Part model, mm, in its own coordinate system. A direction names the side the tool comes from. Round coordinates to 2 decimals unless told otherwise and drop trailing zeros. Write each loop counter-clockwise with the first axis right and the second up, starting at its lowest first coordinate (ties: lowest second). Pieces come first, ordered by that corner, then holes. Notation, with made-up numbers: (-26.5, 61.25) -> (8.5, 61.25) arc R27 cw to (8.5, 91.25) -> close; hole circle Ø10 at (-11, 66). An arc over 180 degrees is marked (long way). Return JSON: item names as keys, results as strings. Group by question number.
```python
from build123d import *

# Parameters (mm, degrees)
BOSS_EXTRUDE1_DEPTH     = 12.88
SWEEP1_START            = 0.63
SWEEP1_DEPTH            = 1.52
LPATTERN1_COUNT         = 3
LPATTERN1_PITCH         = 5
SKETCH5_W               = 2.9
SKETCH5_H               = 0.8
CUT_EXTRUDE1_DEPTH      = 1
LPATTERN2_COUNT         = 2
LPATTERN2_PITCH         = 5.58
MIRROR1_START           = 0.63
MIRROR1_COPY_1_DEPTH    = 1.52
MIRROR1_COPY_2_DEPTH    = 1.52
MIRROR1_COPY_3_SKETCH_W = 2.9
MIRROR1_COPY_3_SKETCH_H = 0.8
MIRROR1_COPY_3_DEPTH    = 1
CUT_EXTRUDE2_REACH      = 21.386
SKETCH6_R               = 1.8
SKETCH7_R               = 2.2
SKETCH7_R_2             = 1.8
BOSS_EXTRUDE2_DEPTH     = 1.4
CUT_EXTRUDE3_DEPTH      = 17.621667755


# Read off the part's stored shape, not the designer's step: Sweep1
with BuildPart() as part:
    # Sketch1 → Boss-Extrude1 (new body)
    with BuildSketch(Plane(origin=(0, 0, 0), x_dir=(0, 0, -1), z_dir=(1, 0, 0))):
        with BuildLine():
            Line((0, 0), (0, 5.15))
            ThreePointArc((0, 5.15), (0.351471863, 5.998528137), (1.2, 6.35))
            Line((1.2, 6.35), (6.7, 6.35))
            ThreePointArc((6.7, 6.35), (7.548528137, 5.998528137), (7.9, 5.15))
            Line((7.9, 5.15), (7.9, 0))
            Line((7.9, 0), (7.1, 0))
            Line((7.1, 0), (7.1, 5.15))
            ThreePointArc((7.1, 5.15), (6.982842712, 5.432842712), (6.7, 5.55))
            Line((6.7, 5.55), (1.2, 5.55))
            ThreePointArc((1.2, 5.55), (0.917157288, 5.432842712), (0.8, 5.15))
            Line((0.8, 5.15), (0.8, 0))
            Line((0.8, 0), (0, 0))
        make_face()
    extrude(amount=BOSS_EXTRUDE1_DEPTH)

    # Sweep1 outline → Sweep1 (add)
    with BuildSketch(Plane.YZ.offset(SWEEP1_START)):
        with BuildLine():
            add(Edge.make_bspline(
                [(-0.846283759, -8.124029358), (-0.858016898, -8.129757785), (-0.870152204, -8.135642842), (-1.003345202, -8.19967658), (-1.15196737, -8.253874655), (-1.433217357, -8.328196696), (-1.577221625, -8.352525408), (-2.012213537, -8.385830326), (-2.305250753, -8.352541538), (-2.584692284, -8.272379972)],
                knots=[-0.008659355, -0.008659355, -0.008659355, -0.008659355, 0, 0, 0.081660017, 0.081660017, 0.163320034, 0.163320034, 0.326640068, 0.326640068, 0.326640068, 0.326640068], degree=3))
            ThreePointArc((-0.846283759, -8.124029358), (-0.431086788, -7.982015265), (0, -7.9))
            Line((0, -7.9), (0, -7.1))
            add(Edge.make_bspline(
                [(0, -7.1), (-0.377073857, -7.135252748), (-0.796992874, -7.239007705), (-1.153651992, -7.390208706), (-1.166116228, -7.395524363), (-1.178338095, -7.400759688)],
                knots=[0, 0, 0, 0, 1, 1, 1.037382886, 1.037382886, 1.037382886, 1.037382886], degree=3))
            ThreePointArc((-1.178338095, -7.400759688), (-1.724000867, -7.564826814), (-2.292574798, -7.527620028))
            Line((-2.292574798, -7.527620028), (-5.183941257, -6.727620028))
            Line((-5.183941257, -6.727620028), (-5.476058743, -7.472379972))
            Line((-5.476058743, -7.472379972), (-2.584692284, -8.272379972))
        make_face()
    sweep1 = extrude(amount=SWEEP1_DEPTH)

    # LPattern1: Sweep1 ×3
    with Locations(*[(i * LPATTERN1_PITCH, 0, 0) for i in range(1, LPATTERN1_COUNT)]):
        add(sweep1)

    # Sketch5 → Cut-Extrude1 (cut)
    with BuildSketch(Plane.XZ):
        with Locations((3.6, -7.5)):
            Rectangle(SKETCH5_W, SKETCH5_H)
    cut_extrude1 = extrude(amount=-CUT_EXTRUDE1_DEPTH, mode=Mode.SUBTRACT)

    # LPattern2: Cut-Extrude1 ×2
    with Locations(*[(i * LPATTERN2_PITCH, 0, 0) for i in range(1, LPATTERN2_COUNT)]):
        add(cut_extrude1, mode=Mode.SUBTRACT)

    # Mirror1: Sweep1, Cut-Extrude1 across plane
    add(sweep1.mirror(Plane(origin=(0, 0, -3.95), x_dir=(1, 0, 0), z_dir=(0, 0, -1))))
    add(cut_extrude1.mirror(Plane(origin=(0, 0, -3.95), x_dir=(1, 0, 0), z_dir=(0, 0, -1))), mode=Mode.SUBTRACT)

    # Mirror1 copy 1 sketch → Mirror1 copy 1 (add)
    with BuildSketch(Plane(origin=(5, 0, -7.9), x_dir=(0, 1, 0), z_dir=(1, 0, 0)).offset(MIRROR1_START)):
        with BuildLine():
            add(Edge.make_bspline(
                [(-0.846283759, 8.124029358), (-0.858016898, 8.129757785), (-0.870152204, 8.135642842), (-1.003345202, 8.19967658), (-1.15196737, 8.253874655), (-1.433217357, 8.328196696), (-1.577221625, 8.352525408), (-2.012213537, 8.385830326), (-2.305250753, 8.352541538), (-2.584692284, 8.272379972)],
                knots=[-0.008659355, -0.008659355, -0.008659355, -0.008659355, 0, 0, 0.081660017, 0.081660017, 0.163320034, 0.163320034, 0.326640068, 0.326640068, 0.326640068, 0.326640068], degree=3))
            ThreePointArc((-0.846283759, 8.124029358), (-0.431086788, 7.982015265), (0, 7.9))
            Line((0, 7.9), (0, 7.1))
            add(Edge.make_bspline(
                [(0, 7.1), (-0.377073857, 7.135252748), (-0.796992874, 7.239007705), (-1.153651992, 7.390208706), (-1.166116228, 7.395524363), (-1.178338095, 7.400759688)],
                knots=[0, 0, 0, 0, 1, 1, 1.037382886, 1.037382886, 1.037382886, 1.037382886], degree=3))
            ThreePointArc((-1.178338095, 7.400759688), (-1.724000867, 7.564826814), (-2.292574798, 7.527620028))
            Line((-2.292574798, 7.527620028), (-5.183941257, 6.727620028))
            Line((-5.183941257, 6.727620028), (-5.476058743, 7.472379972))
            Line((-5.476058743, 7.472379972), (-2.584692284, 8.272379972))
        make_face()
    extrude(amount=MIRROR1_COPY_1_DEPTH)

    # Mirror1 copy 2 sketch → Mirror1 copy 2 (add)
    with BuildSketch(Plane(origin=(10, 0, -7.9), x_dir=(0, 1, 0), z_dir=(1, 0, 0)).offset(MIRROR1_START)):
        with BuildLine():
            add(Edge.make_bspline(
                [(-0.846283759, 8.124029358), (-0.858016898, 8.129757785), (-0.870152204, 8.135642842), (-1.003345202, 8.19967658), (-1.15196737, 8.253874655), (-1.433217357, 8.328196696), (-1.577221625, 8.352525408), (-2.012213537, 8.385830326), (-2.305250753, 8.352541538), (-2.584692284, 8.272379972)],
                knots=[-0.008659355, -0.008659355, -0.008659355, -0.008659355, 0, 0, 0.081660017, 0.081660017, 0.163320034, 0.163320034, 0.326640068, 0.326640068, 0.326640068, 0.326640068], degree=3))
            ThreePointArc((-0.846283759, 8.124029358), (-0.431086788, 7.982015265), (0, 7.9))
            Line((0, 7.9), (0, 7.1))
            add(Edge.make_bspline(
                [(0, 7.1), (-0.377073857, 7.135252748), (-0.796992874, 7.239007705), (-1.153651992, 7.390208706), (-1.166116228, 7.395524363), (-1.178338095, 7.400759688)],
                knots=[0, 0, 0, 0, 1, 1, 1.037382886, 1.037382886, 1.037382886, 1.037382886], degree=3))
            ThreePointArc((-1.178338095, 7.400759688), (-1.724000867, 7.564826814), (-2.292574798, 7.527620028))
            Line((-2.292574798, 7.527620028), (-5.183941257, 6.727620028))
            Line((-5.183941257, 6.727620028), (-5.476058743, 7.472379972))
            Line((-5.476058743, 7.472379972), (-2.584692284, 8.272379972))
        make_face()
    extrude(amount=MIRROR1_COPY_2_DEPTH)

    # Mirror1 copy 3 sketch → Mirror1 copy 3 (cut)
    with BuildSketch(Plane(origin=(5.58, 0, -7.9), x_dir=(1, 0, 0), z_dir=(0, -1, 0))):
        with Locations((3.6, 7.5)):
            Rectangle(MIRROR1_COPY_3_SKETCH_W, MIRROR1_COPY_3_SKETCH_H)
    extrude(amount=-MIRROR1_COPY_3_DEPTH, mode=Mode.SUBTRACT)

    # Sketch6 → Cut-Extrude2 (cut, up to next)
    with BuildSketch(Plane(origin=(0, 6.35, 0), x_dir=(1, 0, 0), z_dir=(0, 1, 0)), mode=Mode.PRIVATE) as cut_extrude2_sk1:
        with Locations(Location((6.44, 3.95, 0), (0, 0, 270))):
            Circle(SKETCH6_R)
    cut_extrude2_tool1 = extrude(cut_extrude2_sk1.sketch, amount=-CUT_EXTRUDE2_REACH, mode=Mode.PRIVATE) & part.part
    add(cut_extrude2_tool1.solids().sort_by_distance((6.44, 6.35, -3.95))[0], mode=Mode.SUBTRACT)

    # Sketch7 → Boss-Extrude2 (add)
    with BuildSketch(Plane.XZ.offset(-5.55)):
        with Locations(Location((6.44, -3.95, 0), (0, 0, 90))):
            Circle(SKETCH7_R)
        with Locations(Location((6.44, -3.95, 0), (0, 0, 90))):
            Circle(SKETCH7_R_2, mode=Mode.SUBTRACT)
    extrude(amount=BOSS_EXTRUDE2_DEPTH)

    # Sketch8 → Cut-Extrude3 (cut, through all)
    with BuildSketch(Plane.ZY):
        Polygon((-6.603043073, 6.35), (-6.453043073, 6.2), (-6.303043073, 6.35), align=None)
        Polygon((-5.303043073, 6.35), (-5.603043073, 6.35), (-5.453043073, 6.2), align=None)
        Polygon((-4.303043073, 6.35), (-4.603043073, 6.35), (-4.453043073, 6.2), align=None)
        Polygon((-3.303043073, 6.35), (-3.603043073, 6.35), (-3.453043073, 6.2), align=None)
        Polygon((-2.303043073, 6.35), (-2.603043073, 6.35), (-2.453043073, 6.2), align=None)
        Polygon((-1.303043073, 6.35), (-1.603043073, 6.35), (-1.453043073, 6.2), align=None)
    extrude(amount=-CUT_EXTRUDE3_DEPTH, mode=Mode.SUBTRACT)


solid = part.part
```
Item 1: Two-plate mould, pull along Y, no slides. Class faces 4 (the face through (6.35, 6.008, -7.539)), 5 (the face through (6.379, -4.051, -7.867)), 6 (the face through (6.379, -1.716, -0.336)): released by +Y, released by -Y, zero draft, split by the parting line, or undercut.
Item 2: Cut at B-B (y = 0.5). Write the cut outline in (x, z).
Item 3: Cut at A-A (z = -3.95). Write the cut outline in (x, y), then the cut area to 3 significant figures.
Item 4: Wall check: L1, parallel to X at y = 0.5, z = -7.75; L2, parallel to X at y = -0.25, z = 0; L3, parallel to X at y = 5.9, z = -3.95. Give the ranges that are in metal, low to high.
Item 5: Flat gauge pins, fed straight in: P1, Ø4, axis at x = 3.5, y = 3, coming from the -Z side; P2, Ø2, axis at x = 9, z = -6.5, coming from the -Y side; P3, Ø1.8, axis at y = -2.5, z = -7.5, coming from the +X side. Where does each tip first touch, or does it go through?
Item 6: Cut at C-C (z = -1). Write the cut outline in (x, y).
Item 7: Which spindle directions (+Z, -Z, +X, -X, +Y, -Y) get a long thin tool onto all of the face, cutting with end or side? Do faces 1 (the face through (7.73, 0.5, -7.5)), 2 (the face through (0.63, -3, 0)), 3 (the face through (11.379, -3.718, -7.133)). Say none if no direction does.
Checks:
{
 "1": {"face 4": "released by +Y", "face 5": "released by -Y", "face 6": "undercut"},
 "2": {"outline": "(0, -7.9) -> (2.15, -7.9) -> (2.15, -7.1) -> (0, -7.1) -> close; (0, -0.8) -> (2.15, -0.8) -> (2.15, 0) -> (0, 0) -> close; (5.05, -7.9) -> (7.73, -7.9) -> (7.73, -7.1) -> (5.05, -7.1) -> close; (5.05, -0.8) -> (7.73, -0.8) -> (7.73, 0) -> (5.05, 0) -> close; (10.63, -7.9) -> (12.88, -7.9) -> (12.88, -7.1) -> (10.63, -7.1) -> close; (10.63, -0.8) -> (12.88, -0.8) -> (12.88, 0) -> (10.63, 0) -> close"},
 "3": {"outline": "(0, 5.55) -> (4.24, 5.55) -> (4.24, 4.15) -> (4.64, 4.15) -> (4.64, 6.35) -> (0, 6.35) -> close; (8.24, 4.15) -> (8.64, 4.15) -> (8.64, 5.55) -> (12.88, 5.55) -> (12.88, 6.35) -> (8.24, 6.35) -> close", "area": "8.54 mm2"},
 "4": {"L1": "x = 0 to 2.15, 5.05 to 7.73, 10.63 to 12.88", "L2": "x = 0.63 to 2.15, 5.63 to 7.15, 10.63 to 12.15", "L3": "x = 0 to 4.64, 8.24 to 12.88"},
 "5": {"P1": "stops at z = -7.9", "P2": "stops at y = 1", "P3": "stops at x = 12.15"},
 "6": {"outline": "(0, 5.5) -> (12.88, 5.5) -> (12.88, 6.33) -> (0, 6.33) -> close; (0.63, -5.25) -> (2.15, -5.25) -> (2.15, -4.56) -> (0.63, -4.56) -> close; (5.63, -5.25) -> (7.15, -5.25) -> (7.15, -4.56) -> (5.63, -4.56) -> close; (10.63, -5.25) -> (12.15, -5.25) -> (12.15, -4.56) -> (10.63, -4.56) -> close"},
 "7": {"face 1": "+Z, -Z, -Y", "face 2": "+Z, -Z, -X, -Y", "face 3": "+X, -X"}
}
